Build history of the part. All positions in model axes, mm. Face numbers are marked on the shaded views. A direction names the side the tool comes from. Give positions to 0.01 mm unless a question says otherwise; leave off trailing zeros. Write each loop counter-clockwise with the first axis right and the second up, starting at its lowest first coordinate (ties: lowest second). Pieces come first, ordered by that corner, then holes. Notation, with made-up numbers: M -9.75,37.25 L 39.25,37.25 A20 cw 39.25,67.25 Z; hole C 42,-33.5 d10. An arc over 180 degrees is marked long. Return JSON: item names as keys, results as strings. Group by question number.
Q1. Tool access for the marked faces 1 and 2: list every direction of +Z, -Z, +X, -X, +Y, -Y with a clear straight run to the whole face (end or side of a thin tool).
Q2. Band-saw the part on A-A, the plane x = -2.75. Count the separate pieces of the cut face and the enclosed holes in it, then the cut area to 3 significant figures.
Q3. Wall check: probe 1 along X at (y, z) = (54, 47); probe 2 along Y at (x, z) = (7, -65); probe 3 along Y at (x, z) = (-5.25, 4). Give the ranges that are in metal, low to high.
Q4. Flat gauge pins, fed straight in: pin 1 Ø2 at (x, z) = (13, -32.5) entering from -Y; pin 2 Ø3 at (y, z) = (-52.5, 69.5) entering from -X; pin 3 Ø5 at (x, y) = (0.5, -69) entering from -Z. Where does each tip first touch, or does it go through?
Q5. Band-saw the part on C-C, the plane z = 80. Give the cut face in (x, y), then the cut area to 3 significant figures.
Q6. Band-saw the part on D-D, the plane y = 33.5. Give the cut face in (x, z).
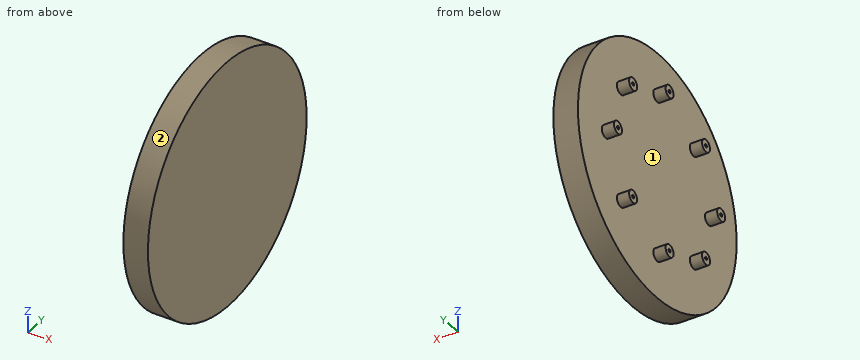
from build123d import *

# Parameters (mm, degrees)
SKETCH1_R           = 100
BOSS_EXTRUDE1_DEPTH = 20
SKETCH4_R           = 1.3
CUT_EXTRUDE2_DEPTH  = 18
BOSS_EXTRUDE3_START = 10
SKETCH5_R           = 5
SKETCH5_R_2         = 1.3
BOSS_EXTRUDE3_DEPTH = 10


with BuildPart() as part:
    # Sketch1 → Boss-Extrude1 (new body)
    with BuildSketch(Plane(origin=(0, 0, 0), x_dir=(0, 0, -1), z_dir=(1, 0, 0))):
        Circle(SKETCH1_R)
    extrude(amount=BOSS_EXTRUDE1_DEPTH)

    # Sketch4 → Cut-Extrude2 (cut)
    with BuildSketch(Plane.ZY):
        with Locations((0, 65)):
            Circle(SKETCH4_R)
        with Locations((45.961940777, 45.961940777)):
            Circle(SKETCH4_R)
        with Locations((65, 0)):
            Circle(SKETCH4_R)
        with Locations((45.961940777, -45.961940777)):
            Circle(SKETCH4_R)
        with Locations((0, -65)):
            Circle(SKETCH4_R)
        with Locations((-45.961940777, -45.961940777)):
            Circle(SKETCH4_R)
        with Locations((-65, 0)):
            Circle(SKETCH4_R)
        with Locations((-45.961940777, 45.961940777)):
            Circle(SKETCH4_R)
    extrude(amount=-CUT_EXTRUDE2_DEPTH, mode=Mode.SUBTRACT)

    # Sketch5 → Boss-Extrude3 (add)
    # profile 1 of 8: a face of its own
    with BuildSketch(Plane.ZY.offset(BOSS_EXTRUDE3_START)):
        with Locations(Location((0, 65, 0), (0, 0, 180))):
            Circle(SKETCH5_R)
        with Locations((0, 65)):
            Circle(SKETCH5_R_2, mode=Mode.SUBTRACT)
    # profile 2 of 8: a face of its own
    with BuildSketch(Plane.ZY.offset(BOSS_EXTRUDE3_START)):
        with Locations(Location((45.961940777, 45.961940777, 0), (0, 0, 180))):
            Circle(SKETCH5_R)
        with Locations((45.961940777, 45.961940777)):
            Circle(SKETCH5_R_2, mode=Mode.SUBTRACT)
    # profile 3 of 8: a face of its own
    with BuildSketch(Plane.ZY.offset(BOSS_EXTRUDE3_START)):
        with Locations(Location((65, 0, 0), (0, 0, 180))):
            Circle(SKETCH5_R)
        with Locations((65, 0)):
            Circle(SKETCH5_R_2, mode=Mode.SUBTRACT)
    # profile 4 of 8: a face of its own
    with BuildSketch(Plane.ZY.offset(BOSS_EXTRUDE3_START)):
        with Locations(Location((45.961940777, -45.961940777, 0), (0, 0, 180))):
            Circle(SKETCH5_R)
        with Locations((45.961940777, -45.961940777)):
            Circle(SKETCH5_R_2, mode=Mode.SUBTRACT)
    # profile 5 of 8: a face of its own
    with BuildSketch(Plane.ZY.offset(BOSS_EXTRUDE3_START)):
        with Locations(Location((0, -65, 0), (0, 0, 180))):
            Circle(SKETCH5_R)
        with Locations((0, -65)):
            Circle(SKETCH5_R_2, mode=Mode.SUBTRACT)
    # profile 6 of 8: a face of its own
    with BuildSketch(Plane.ZY.offset(BOSS_EXTRUDE3_START)):
        with Locations(Location((-45.961940777, -45.961940777, 0), (0, 0, 180))):
            Circle(SKETCH5_R)
        with Locations((-45.961940777, -45.961940777)):
            Circle(SKETCH5_R_2, mode=Mode.SUBTRACT)
    # profile 7 of 8: a face of its own
    with BuildSketch(Plane.ZY.offset(BOSS_EXTRUDE3_START)):
        with Locations(Location((-65, 0, 0), (0, 0, 180))):
            Circle(SKETCH5_R)
        with Locations((-65, 0)):
            Circle(SKETCH5_R_2, mode=Mode.SUBTRACT)
    # profile 8 of 8: a face of its own
    with BuildSketch(Plane.ZY.offset(BOSS_EXTRUDE3_START)):
        with Locations(Location((-45.961940777, 45.961940777, 0), (0, 0, 180))):
            Circle(SKETCH5_R)
        with Locations((-45.961940777, 45.961940777)):
            Circle(SKETCH5_R_2, mode=Mode.SUBTRACT)
    extrude(amount=-BOSS_EXTRUDE3_DEPTH)


solid = part.part
From the geometry:
{
 "1": {"face 1": "-X", "face 2": "+X, -X"},
 "2": {"separate pieces": "8", "enclosed holes": "8", "area": "586 mm^2"},
 "3": {"probe 1": "x = 0 to 20", "probe 2": "y = -75.99 to -1.3, 1.3 to 75.99", "probe 3": "y = -68 to -62, 62 to 68"},
 "4": {"pin 1": "stops at y = -94.91", "pin 2": "stops at x = 0", "pin 3": "stops at z = -74.68"},
 "5": {"outline": "M 0,-60 L 20,-60 L 20,60 L 0,60 Z", "area": "2,400 mm^2"},
 "6": {"outline": "M 0,-94.22 L 20,-94.22 L 20,94.22 L 0,94.22 Z"}
}
